Design review of the part built by this model. Coordinates are the model's own, in mm. Give positions to 0.01 mm unless a question says otherwise; leave off trailing zeros. Write each loop counter-clockwise with the first axis right and the second up, starting at its lowest first coordinate (ties: lowest second). Pieces come first, ordered by that corner, then holes. Notation, with made-up numbers: (50, 57.25) - (90, 57.25) arc R27 ccw to (90, 95.25) - close; hole circle Ø1 at (75, 0.5). An arc over 180 degrees is marked (long way). Use a Markdown table: item, result. Add a question column.
```python
from build123d import *

# Parameters (mm, degrees)
SKETCH_2_W          = 5
SKETCH_2_H          = 13
SKETCH_4_R          = 1.25
CUT_EXTRUDE_1_DEPTH = 20.209372712


with BuildPart() as part:
    # 草图2 → 旋转1 (revolve)
    with BuildSketch(Plane.XY, mode=Mode.PRIVATE) as revolve_1_sk:
        with Locations((7.5, 6.5)):
            Rectangle(SKETCH_2_W, SKETCH_2_H)
    revolve(revolve_1_sk.sketch.rotate(Axis((0, 13, 0), (0, -1, 0)), 180), axis=Axis((0, 13, 0), (0, -1, 0)))

    # 草图4 → 切除-拉伸1 (cut, through all)
    with BuildSketch(Plane(origin=(0, 13, 0), x_dir=(1, 0, 0), z_dir=(0, 1, 0))):
        with Locations(Location((0, 7.5, 0), (0, 0, 270))):
            Circle(SKETCH_4_R)
        with Locations(Location((7.5, 0, 0), (0, 0, 270))):
            Circle(SKETCH_4_R)
        with Locations(Location((0, -7.5, 0), (0, 0, 270))):
            Circle(SKETCH_4_R)
        with Locations(Location((-7.5, 0, 0), (0, 0, 270))):
            Circle(SKETCH_4_R)
    extrude(amount=-CUT_EXTRUDE_1_DEPTH, mode=Mode.SUBTRACT)


solid = part.part
```
(1) For line 1 along X through (y, z) = (5, 1); line 2 along Z through (x, y) = (-4.25, 11.25); line 3 along X through (y, z) = (10.5, 1.5), list the stretches that pass through material, from the lowest coordinate up.
(2) Add section B-B (x = -1.5). State the section outline as (y, z) points, and give its area (3 significant figures).
(3) Insertion check: pin 1 (4 mm diameter, centred on x = 0, z = -7.5, fed in from +Y); pin 2 (3 mm diameter, centred on x = 5, y = 1.5, fed in from -Z); pin 3 (1.5 mm diameter, centred on y = 6.5, z = 6, fed in from -X); pin 4 (2 mm diameter, centred on x = -7.5, z = 0, fed in from -Y). Each pin has a flat end and moves straight along its axis. Give the tip position at first contact, or say it passes through.
(4) Add section A-A (z = 0). State the section outline as (x, y) points, and give its area (3 significant figures).
(5) Add section C-C (y = 11.75). State the section outline as (x, z) points, and give its area (3 significant figures).
(6) Mouldability with a two-part tool opening along X and no side actions: class faces 1 (the face through (10, 7, 0)), 2 (the face through (2, 13, -5)), 3 (the face through (-8.72, 6.59, -0.27)) as +X half, -X half, draft (parallel to the pull), parting line (faces both ways), or undercut.
(7) Add section D-D (z = 3.5). State the section outline as (x, y) points, and give its area (3 significant figures).
Answers follow:
| question | item | result |
|---|---|---|
| 1 | line 1 | -9.95 to -8.25, -6.75 to -4.9, 4.9 to 6.75, 8.25 to 9.95 |
| 1 | line 2 | -9.05 to -2.63, 2.63 to 9.05 |
| 1 | line 3 | -9.89 to -4.77, 4.77 to 9.89 |
| 2 | outline | (0, -9.89) - (13, -9.89) - (13, -4.77) - (0, -4.77) - close; (0, 4.77) - (13, 4.77) - (13, 9.89) - (0, 9.89) - close |
| 2 | area | 133 mm^2 |
| 3 | pin 1 | y = 13 |
| 3 | pin 2 | z = -9.37 |
| 3 | pin 3 | x = -8.51 |
| 3 | pin 4 | through |
| 4 | outline | (-10, 0) - (-8.75, 0) - (-8.75, 13) - (-10, 13) - close; (-6.25, 0) - (-5, 0) - (-5, 13) - (-6.25, 13) - close; (5, 0) - (6.25, 0) - (6.25, 13) - (5, 13) - close; (8.75, 0) - (10, 0) - (10, 13) - (8.75, 13) - close |
| 4 | area | 65.0 mm^2 |
| 5 | outline | circle Ø20 at (0, 0); hole circle Ø2.5 at (-7.5, 0); hole circle Ø10 at (0, 0); hole circle Ø2.5 at (0, -7.5); hole circle Ø2.5 at (0, 7.5); hole circle Ø2.5 at (7.5, 0) |
| 5 | area | 216 mm^2 |
| 6 | face 1 | parting line |
| 6 | face 2 | draft |
| 6 | face 3 | undercut |
| 7 | outline | (-9.37, 0) - (-3.57, 0) - (-3.57, 13) - (-9.37, 13) - close; (3.57, 0) - (9.37, 0) - (9.37, 13) - (3.57, 13) - close |
| 7 | area | 151 mm^2 |
